Read the model definition and answer for the solid it produces. Units are mm, in the model's axes. Face numbers are marked on the shaded views. Round coordinates to 2 decimals unless told otherwise and drop trailing zeros. Write each loop counter-clockwise with the first axis right and the second up, starting at its lowest first coordinate (ties: lowest second). Pieces come first, ordered by that corner, then holes. Notation, with made-up numbers: (13, 77) -> (50, 77) arc R28 cw to (50, 115) -> close; hole circle Ø11 at (21.25, -6.5). An arc over 180 degrees is marked (long way). Return JSON: item names as keys, results as strings.
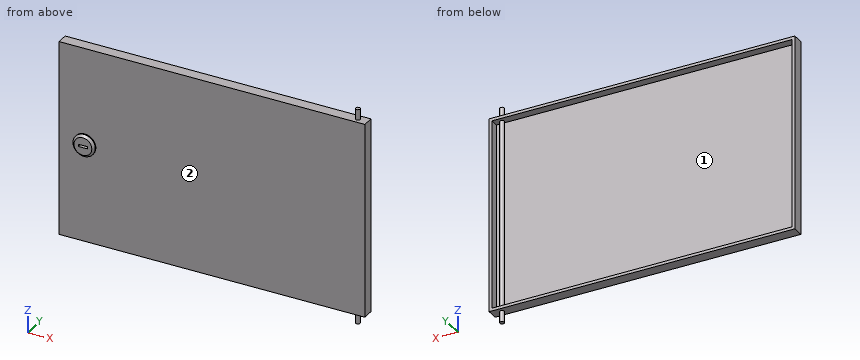
from build123d import *

# Parameters (mm, degrees)
F0_W          = 274.5
F0_H          = 10
F1_DEPTH      = 175.5
F2_T          = -2.5
F3_R          = 2
F4_DEPTH      = 10
F4_DEPTH_BACK = 185
F5_R          = 10
F5_W          = 8
F5_H          = 2
F6_DEPTH      = 3
F7_SIZE       = 2


with BuildPart() as f1:
    # F0 (on Top) → F1 (new body)
    with BuildSketch(Plane.XY):
        with Locations((137.25, 5)):
            Rectangle(F0_W, F0_H)
    extrude(amount=F1_DEPTH)

    # F2
    f2_openings = [f1.faces().sort_by_distance(p)[0] for p in [
        (137.25, 10, 87.75),
    ]]
    offset(amount=F2_T, openings=f2_openings)

    # F3 (on face) → F4 (join, two sides)
    with BuildSketch(Plane(origin=(0, 0, 0), x_dir=(1, 0, 0), z_dir=(0, 0, -1))) as f4_sk:
        with Locations((265.5, -5)):
            Circle(F3_R)
    extrude(amount=F4_DEPTH)
    extrude(f4_sk.sketch, amount=-F4_DEPTH_BACK)

    # F5 (on face) → F6 (join)
    with BuildSketch(Plane.XZ):
        with Locations((22.982316, 87.75)):
            Circle(F5_R)
        with Locations((22.982316, 87.75)):
            Rectangle(F5_W, F5_H, mode=Mode.SUBTRACT)
    extrude(amount=F6_DEPTH)

    # F7
    f7_edges = [f1.edges().sort_by_distance(p)[0] for p in [
        (12.982316, -3, 87.75),
    ]]
    chamfer(f7_edges, length=F7_SIZE)


solid = f1.part
Item 1: Section A-A (z = 71) is taken. Give the vertices of the cut face in (x, y).
Worked answers:
{"outline": "(0, 0) -> (274.5, 0) -> (274.5, 10) -> (272, 10) -> (272, 2.5) -> (2.5, 2.5) -> (2.5, 10) -> (0, 10) -> close; circle Ø4 at (265.5, 5)"}
Item 2: Section B-B (y = 5) is taken. Give the vertices of the cut face in (x, z).
Worked answers:
{"outline": "(0, 0) -> (263.5, 0) -> (263.5, -10) -> (267.5, -10) -> (267.5, 0) -> (274.5, 0) -> (274.5, 175.5) -> (267.5, 175.5) -> (267.5, 185) -> (263.5, 185) -> (263.5, 175.5) -> (0, 175.5) -> close; hole (2.5, 2.5) -> (263.5, 2.5) -> (263.5, 173) -> (2.5, 173) -> close; hole (267.5, 2.5) -> (272, 2.5) -> (272, 173) -> (267.5, 173) -> close"}
Item 3: Section C-C (x = 64) is taken. Give the vertices of the cut face in (y, z), then the cut area to 3 significant figures.
Worked answers:
{"outline": "(0, 0) -> (10, 0) -> (10, 2.5) -> (2.5, 2.5) -> (2.5, 173) -> (10, 173) -> (10, 175.5) -> (0, 175.5) -> close", "area": "476 mm2"}
Item 4: Straight lines are drawn through the part: L1, parallel to X at y = 5.5, z = 28.5; L2, parallel to X at y = 8, z = 87; L3, parallel to Z at x = 203.5, y = 7.5. For each, find the intervals that lie inside material, in ascending order. Write a range as [from, to].
Worked answers:
{"L1": "x = [0, 2.5], [263.56, 267.44], [272, 274.5]", "L2": "x = [0, 2.5], [272, 274.5]", "L3": "z = [0, 2.5], [173, 175.5]"}
Item 5: Flat-ended cylindrical pins translate along their axes: pin 1 (2.5 mm diameter, centred on x = 24.5, y = -1.5, fed in from -Z); pin 2 (1.6 mm diameter, centred on y = -1.5, z = 87.5, fed in from -X); pin 3 (8 mm diameter, centred on x = 64.5, z = 22.5, fed in from +Y). Find the tip coordinate at first contact, or state that the pin passes through.
Worked answers:
{"pin 1": "stops at z = 77.76", "pin 2": "stops at x = 12.98", "pin 3": "stops at y = 2.5"}
Item 6: For a pull along X with two mould halves and no side action, classify the marked faces 1 and 2 as released by +X, released by -X, zero draft, split by the parting line, or undercut.
Worked answers:
{"face 1": "undercut", "face 2": "zero draft"}
